```python
from build123d import *

# Parameters (mm, degrees)
SKETCH1_W           = 115
SKETCH1_H           = 90
BOSS_EXTRUDE1_DEPTH = 5
SKETCH2_W           = 108
SKETCH2_H           = 83.2
BOSS_EXTRUDE2_DEPTH = 3
FILLET1_R           = 5
SKETCH3_W           = 4
SKETCH3_H           = 20
CUT_EXTRUDE1_DEPTH  = 10
FILLET2_R           = 1
SKETCH4_R           = 5
CUT_EXTRUDE2_DEPTH  = 10
FILLET3_R           = 1


with BuildPart() as part:
    # Sketch1 → Boss-Extrude1 (new body)
    with BuildSketch(Plane(origin=(0, 0, 0), x_dir=(1, 0, 0), z_dir=(0, 1, 0))):
        Rectangle(SKETCH1_W, SKETCH1_H)
    extrude(amount=BOSS_EXTRUDE1_DEPTH)

    # Sketch2 → Boss-Extrude2 (add)
    with BuildSketch(Plane(origin=(0, 5, 0), x_dir=(1, 0, 0), z_dir=(0, 1, 0))):
        Rectangle(SKETCH2_W, SKETCH2_H)
    extrude(amount=BOSS_EXTRUDE2_DEPTH)

    # Fillet1
    fillet1_edges = [part.edges().sort_by_distance(p)[0] for p in [
        (57.5, 2.5, 45),
        (-57.5, 2.5, 45),
        (-57.5, 2.5, -45),
        (57.5, 2.5, -45),
    ]]
    fillet(fillet1_edges, radius=FILLET1_R)

    # Sketch3 → Cut-Extrude1 (cut)
    with BuildSketch(Plane(origin=(0, 0, 0), x_dir=(-1, 0, 0), z_dir=(0, -1, 0))):
        with Locations((-49, -24)):
            Rectangle(SKETCH3_W, SKETCH3_H)
    extrude(amount=-CUT_EXTRUDE1_DEPTH, mode=Mode.SUBTRACT)

    # Fillet2
    fillet2_edges = [part.edges().sort_by_distance(p)[0] for p in [
        (47, 0, 24),
        (49, 0, 14),
        (51, 0, 24),
        (49, 0, 34),
    ]]
    fillet(fillet2_edges, radius=FILLET2_R)

    # Sketch4 → Cut-Extrude2 (cut)
    with BuildSketch(Plane.XZ):
        with Locations((47.5, -11)):
            Circle(SKETCH4_R)
    extrude(amount=-CUT_EXTRUDE2_DEPTH, mode=Mode.SUBTRACT)

    # Fillet3
    fillet3_edges = [part.edges().sort_by_distance(p)[0] for p in [
        (42.5, 0, -11),
    ]]
    fillet(fillet3_edges, radius=FILLET3_R)


solid = part.part
```
The listing builds one solid part. Answer for the finished solid, in the listing's coordinates (mm). A direction names the side the tool comes from. Give positions to 0.01 mm unless a question says otherwise; leave off trailing zeros. Order: outer loops, then holes, each group sorted by start corner. A loop starts at its lowest first (then second) coordinate and runs counter-clockwise, first axis right, second up. Notation, with made-up numbers: (10, 26.25) - (46, 26.25) arc R9 ccw to (46, 38.25) - close; hole circle Ø9 at (80.5, 65). An arc over 180 degrees is marked (long way). Answer in a Markdown table with one row per item. Add a question column.
Q1. Find the intervals of material crossed by line 1 along Z through (x, y) = (47.5, 3.25); line 2 along Z through (x, y) = (47.5, 6); line 3 along X through (y, z) = (1.5, 15.5), in increasing order. Write a range as [from, to].
Q2. The part is cut by section D-D (z = 25.5). Determine the outline of the cut face in (x, y), then the cut area to 3 significant figures.
Q3. The part is cut by section A-A (z = -11). Determine the outline of the cut face in (x, y), then the cut area to 3 significant figures.
Q4. The part is cut by section C-C (x = 27). Determine the outline of the cut face in (y, z), then the cut area to 3 significant figures.
Q5. Given P1, Ø2.5, axis at y = 7, z = 17, coming from the -X side; P2, Ø3.5, axis at y = 7, z = 18.5, coming from the +X side; P3, Ø0.9, axis at x = 24, y = 6.5, coming from the -Z side; P4, Ø8, axis at x = 47.5, z = -11, coming from the -Y side, each flat-ended and moving along its own axis, determine where each tip first touches the part or whether it passes through.
Q6. For a pull along Z with two mould halves and no side action, classify faces 1 (the flat face through (49, 4, 14)), 2 (the flat face through (49, 4, 34)), 3 (the flat face through (-1, 2, 45)), 4 (the flat face through (-1, 0, -1)) as released by +Z, released by -Z, zero draft, split by the parting line, or undercut.
Q7. The part is cut by section B-B (y = 3.75). Determine the outline of the cut face in (x, z), then the cut area to 3 significant figures.
Q8. Which of the six approach directions +Z, -Z, +X, -X, +Y, -Y give full straight-line access (tool end or side, diameter ignored) to faces 5 (the flat face through (47, 4, 24)), 6 (the flat face through (-1, 6, 41.6)), 7 (the flat face through (-1, 6, -41.6))?
Determined:
| question | item | result |
|---|---|---|
| 1 | line 1 | z = [-45, -16], [-6, 14], [34, 45] |
| 1 | line 2 | z = [-41.6, -16], [-6, 14], [34, 41.6] |
| 1 | line 3 | x = [-57.5, 47], [51, 57.5] |
| 2 | outline | (-57.5, 0) - (46, 0) arc R1 ccw to (47, 1) - (47, 8) - (-54, 8) - (-54, 5) - (-57.5, 5) - close; (51, 1) arc R1 ccw to (52, 0) - (57.5, 0) - (57.5, 5) - (54, 5) - (54, 8) - (51, 8) - close |
| 2 | area | 867 mm² |
| 3 | outline | (-57.5, 0) - (41.5, 0) arc R1 ccw to (42.5, 1) - (42.5, 8) - (-54, 8) - (-54, 5) - (-57.5, 5) - close; (52.5, 1) arc R1 ccw to (53.5, 0) - (57.5, 0) - (57.5, 5) - (54, 5) - (54, 8) - (52.5, 8) - close |
| 3 | area | 819 mm² |
| 4 | outline | (0, -45) - (5, -45) - (5, -41.6) - (8, -41.6) - (8, 41.6) - (5, 41.6) - (5, 45) - (0, 45) - close |
| 4 | area | 700 mm² |
| 5 | P1 | stops at x = -54 |
| 5 | P2 | stops at x = 54 |
| 5 | P3 | stops at z = -41.6 |
| 5 | P4 | passes through |
| 6 | face 1 | undercut |
| 6 | face 2 | undercut |
| 6 | face 3 | released by +Z |
| 6 | face 4 | zero draft |
| 7 | outline | (-57.5, -40) arc R5 ccw to (-52.5, -45) - (52.5, -45) arc R5 ccw to (57.5, -40) - (57.5, 40) arc R5 ccw to (52.5, 45) - (-52.5, 45) arc R5 ccw to (-57.5, 40) - close; hole circle Ø10 at (47.5, -11); hole (47, 14) - (51, 14) - (51, 34) - (47, 34) - close |
| 7 | area | 10,200 mm² |
| 8 | face 5 | +Y, -Y |
| 8 | face 6 | +Z, +X, -X, +Y |
| 8 | face 7 | -Z, +X, -X, +Y |
